Verification items for this drawing (mm, ordinates from the low corner). Coordinates: 2 decimals unless noted, no trailing zeros. Write each loop counter-clockwise with the first axis right and the second up, starting at its lowest first coordinate (ties: lowest second). Pieces come first, ordered by that corner, then holes. Notation, with made-up numbers: (12, 41.25) -> (55, 41.25) arc R24 cw to (55, 67.25) -> close; hole circle Ø4 at (6, -28.75). An arc over 180 degrees is marked (long way). Use CSV: the item, a comma, the result in double quotes.
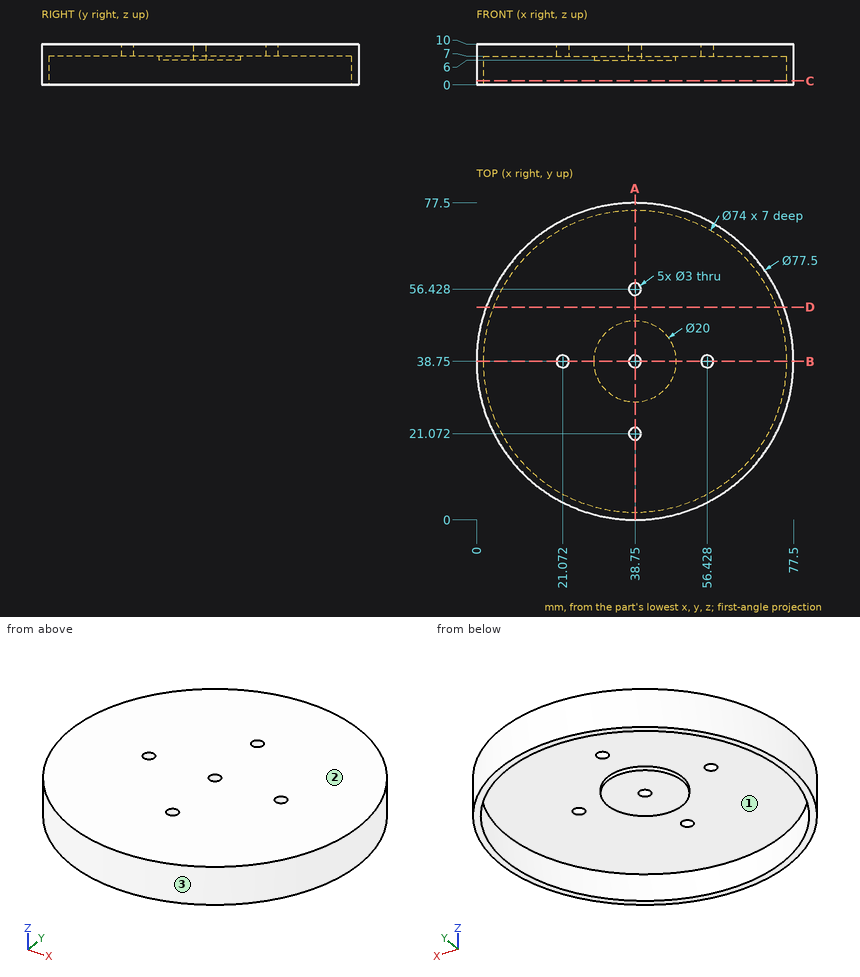
1) Scan lines: L1, parallel to Y at x = 38.75, z = 8.65; L2, parallel to Y at x = 38.75, z = 5.25; L3, parallel to Z at x = 58.5, y = 25.5. Record each from-to range of solid material in increasing order.
Return value:
L1,"0 to 19.57, 22.57 to 37.25, 40.25 to 54.93, 57.93 to 77.5"
L2,"0 to 1.75, 75.75 to 77.5"
L3,"7 to 10"
2) Gauge pin test, flat ends, axial feed: pin 1 (6 mm diameter, centred on y = 60.5, z = 5.5, fed in from +X); pin 2 (1.5 mm diameter, centred on x = 26, z = 6.5, fed in from -Y) (1 decimal); pin 3 (2 mm diameter, centred on x = 13, z = 2, fed in from +Y) (1 decimal). Record the tip position at first contact, or that the pin passes through.
Return value:
pin 1,"x = 72.66"
pin 2,"y = 1.9"
pin 3,"y = 68.6"
3) Cross-section at C-C (z = 1). Record the boundary of the cut face in (x, y).
Return value:
outline,"circle Ø77.5 at (38.75, 38.75); hole circle Ø74 at (38.75, 38.75)"
4) Cross-section at D-D (y = 52). Record the boundary of the cut face in (x, z), plus the area to 3 significant figures.
Return value:
outline,"(2.34, 0) -> (4.2, 0) -> (4.2, 7) -> (73.3, 7) -> (73.3, 0) -> (75.16, 0) -> (75.16, 10) -> (2.34, 10) -> close"
area,"245 mm2"
5) Mould release check, pull along X, two halves, no side actions. Record for the marked faces 1, 2 and 3: released by +X, released by -X, zero draft, split by the parting line, or undercut.
Return value:
face 1,"undercut"
face 2,"zero draft"
face 3,"split by the parting line"
6) Cross-section at A-A (x = 38.75). Record the boundary of the cut face in (y, z), plus the area to 3 significant figures.
Return value:
outline,"(0, 0) -> (1.75, 0) -> (1.75, 7) -> (19.57, 7) -> (19.57, 10) -> (0, 10) -> close; (22.57, 7) -> (28.75, 7) -> (28.75, 6) -> (37.25, 6) -> (37.25, 10) -> (22.57, 10) -> close; (40.25, 6) -> (48.75, 6) -> (48.75, 7) -> (54.93, 7) -> (54.93, 10) -> (40.25, 10) -> close; (57.93, 7) -> (75.75, 7) -> (75.75, 0) -> (77.5, 0) -> (77.5, 10) -> (57.93, 10) -> close"
area,"247 mm2"
